```python
from build123d import *

# Parameters (mm, degrees)
EXTRUSION1_DEPTH = 49.5
ESQUISSE2_R      = 1.5
ESQUISSE2_W      = 18.5
ESQUISSE2_H      = 20
EXTRUSION2_DEPTH = 100
ESQUISSE3_R      = 1.5
EXTRUSION3_DEPTH = 100


with BuildPart() as part:
    # Esquisse1 → Extrusion1 (new body)
    with BuildSketch(Plane.XY):
        Polygon((-24.93137059, 6.591473684), (-24.93137059, -13.408526316), (-4.93137059, -13.408526316), (-4.93137059, -11.908526316), (-23.43137059, -11.908526316), (-23.43137059, 6.591473684), align=None)
    extrude(amount=EXTRUSION1_DEPTH)

    # Esquisse2 → Extrusion2 (cut)
    with BuildSketch(Plane(origin=(0, -11.908526316, 0), x_dir=(-1, 0, 0), z_dir=(0, 1, 0))):
        with Locations((14.93137059, 43.5)):
            Circle(ESQUISSE2_R)
        with Locations((14.93137059, 30)):
            Circle(ESQUISSE2_R)
        with Locations((14.18137059, 10)):
            Rectangle(ESQUISSE2_W, ESQUISSE2_H)
    extrude(amount=-EXTRUSION2_DEPTH, mode=Mode.SUBTRACT)

    # Esquisse3 → Extrusion3 (cut)
    with BuildSketch(Plane(origin=(-23.43137059, 0, 0), x_dir=(0, 0, -1), z_dir=(1, 0, 0))):
        with Locations((-11.5, -3.408526316)):
            Circle(ESQUISSE3_R)
    extrude(amount=-EXTRUSION3_DEPTH, mode=Mode.SUBTRACT)


solid = part.part
```
The listing builds one solid part. Answer for the finished solid, in the listing's coordinates (mm). A direction names the side the tool comes from. Coordinates: 2 decimals unless noted, no trailing zeros. Write each loop counter-clockwise with the first axis right and the second up, starting at its lowest first coordinate (ties: lowest second). Pieces come first, ordered by that corner, then holes.
Q1. Section B-B, the plane x = -15.25 is taken. Write down the section's boundary in (y, z), then the cut area to 3 significant figures.
Returned:
outline: (-13.41, 20) - (-11.91, 20) - (-11.91, 28.53) - (-13.41, 28.53) - close; (-13.41, 31.47) - (-11.91, 31.47) - (-11.91, 42.03) - (-13.41, 42.03) - close; (-13.41, 44.97) - (-11.91, 44.97) - (-11.91, 49.5) - (-13.41, 49.5) - close
area: 35.5 mm2
Q2. Section A-A, the plane z = 30 is taken. Write down the section's boundary in (x, y).
Returned:
outline: (-24.93, -13.41) - (-16.43, -13.41) - (-16.43, -11.91) - (-23.43, -11.91) - (-23.43, 6.59) - (-24.93, 6.59) - close; (-13.43, -13.41) - (-4.93, -13.41) - (-4.93, -11.91) - (-13.43, -11.91) - close
Q3. Find the intervals of material crossed by line 1 along Y through (x, z) = (-6.5, 39.5); line 2 along Y through (x, z) = (-24, 11.5); line 3 along X through (y, z) = (2.25, 27), in increasing order.
Returned:
line 1: y = -13.41 to -11.91
line 2: y = -13.41 to -4.91, -1.91 to 6.59
line 3: x = -24.93 to -23.43
Q4. Which of the six approach directions +Z, -Z, +X, -X, +Y, -Y give full straight-line access (tool end or side, diameter ignored) to faces 5 (the flat face through (-15, -13.409, 35)), 6 (the flat face through (-14, -11.909, 35))?
Returned:
face 5: +Z, -Z, +X, -X, -Y
face 6: +Z, -Z, +X, +Y
Q5. Given P1, Ø4, axis at y = -3.41, z = 11.5, coming from the -X side; P2, Ø6, axis at y = -6.5, z = 23.5, coming from the +X side; P3, Ø5, axis at x = -14.93, z = 30, coming from the +Y side, each flat-ended and moving along its own axis, determine where each tip first touches the part or whether it passes through.
Returned:
P1: stops at x = -24.93
P2: stops at x = -23.43
P3: stops at y = -11.91
Q6. Section C-C, the plane y = -10.75 is taken. Write down the section's boundary in (x, z).
Returned:
outline: (-24.93, 0) - (-23.43, 0) - (-23.43, 49.5) - (-24.93, 49.5) - close
Q7. The mould has two halves that part along Z. Classify faces 1 (the cylindrical face through (-15, -13, 42)), 2 (the cylindrical face through (-13.826, -12.648, 31.014)), 3 (the flat face through (-14, -13, 20)), 4 (the flat face through (-24, 6.591, 24)): released by +Z, released by -Z, zero draft, split by the parting line, or undercut.
Returned:
face 1: undercut
face 2: undercut
face 3: released by -Z
face 4: zero draft
Q8. Section D-D, the plane z = 11.5 is taken. Write down the section's boundary in (x, y), then the cut area to 3 significant figures.
Returned:
outline: (-24.93, -13.41) - (-23.43, -13.41) - (-23.43, -4.91) - (-24.93, -4.91) - close; (-24.93, -1.91) - (-23.43, -1.91) - (-23.43, 6.59) - (-24.93, 6.59) - close
area: 25.5 mm2
